Source: CAD feature listing. Evaluate the final solid. Frame: model axes, mm. Coordinates: 2 decimals unless noted, no trailing zeros. Order: outer loops, then holes, each group sorted by start corner. A loop starts at its lowest first (then second) coordinate and runs counter-clockwise, first axis right, second up.
```python
from build123d import *

# Parameters (mm, degrees)
F1_DEPTH    = 3
F2_T1_DEPTH = 3


# Not quite as in the source:
# - a fillet or chamfer that OpenCascade refuses, or shapes differently, is made with other operations: its cross-section is extruded or revolved along the edge and cut away or added


with BuildPart() as f1:
    # F0 (on Front) → F1 (new body)
    with BuildSketch(Plane.XZ):
        with BuildLine():
            Line((-12.6923788449, -38.0739606037), (-14.2292520278, -43.8096494069))
            ThreePointArc((-14.2292520278, -43.8096494069), (-12.3693152355, -44.4080485447), (-10.4843489922, -44.9221970263))
            ThreePointArc((-10.4843489922, -44.9221970263), (-10.6097140662, -41.870019803), (-7.9435705793, -43.3610533745))
            ThreePointArc((-7.9435705793, -43.3610533745), (-8.4561337122, -44.5984902415), (-9.6935705793, -45.1110533745))
            ThreePointArc((-9.6935705793, -45.1110533745), (-7.8201224186, -45.4967770693), (-5.9315086401, -45.7996446565))
            Line((-5.9315086401, -45.7996446565), (-4.35, -39.8973740589))
            ThreePointArc((-4.35, -39.8973740589), (-8.5698237047, -39.2081761686), (-12.6923788449, -38.0739606037))
        make_face()
        with BuildLine():
            Line((-14.2292520278, -43.8096494069), (-14.9257175554, -46.4088941417))
            ThreePointArc((-14.9257175554, -46.4088941417), (-10.8052141087, -47.537457316), (-6.6017256924, -48.3009287476))
            Line((-6.6017256924, -48.3009287476), (-5.9315086401, -45.7996446565))
            ThreePointArc((-5.9315086401, -45.7996446565), (-7.8201224186, -45.4967770693), (-9.6935705793, -45.1110533745))
            ThreePointArc((-9.6935705793, -45.1110533745), (-10.1000792565, -45.063184596), (-10.4843489922, -44.9221970263))
            ThreePointArc((-10.4843489922, -44.9221970263), (-12.3693152355, -44.4080485447), (-14.2292520278, -43.8096494069))
        make_face()
        with BuildLine():
            ThreePointArc((14.9257175554, -46.4088941417), (39.3966447228, -28.7135313848), (48.75, 0))
            ThreePointArc((48.75, 0), (-28.7135313848, 39.3966447228), (-14.9257175554, -46.4088941417))
            Line((-14.9257175554, -46.4088941417), (-14.2292520278, -43.8096494069))
            ThreePointArc((-14.2292520278, -43.8096494069), (-25.1843873236, 32.6155595225), (43.434381424, -2.7721802304))
            ThreePointArc((43.434381424, -2.7721802304), (35.3877397529, -27.956567554), (14.2292520278, -43.8096494069))
            Line((14.2292520278, -43.8096494069), (14.9257175554, -46.4088941417))
        make_face()
        with BuildLine():
            ThreePointArc((10.4843489922, -44.9221970263), (12.3693152355, -44.4080485447), (14.2292520278, -43.8096494069))
            Line((14.2292520278, -43.8096494069), (12.6923788449, -38.0739606037))
            ThreePointArc((12.6923788449, -38.0739606037), (8.5698237047, -39.2081761686), (4.35, -39.8973740589))
            Line((4.35, -39.8973740589), (5.9315086401, -45.7996446565))
            ThreePointArc((5.9315086401, -45.7996446565), (7.8201224186, -45.4967770693), (9.6935705793, -45.1110533745))
            ThreePointArc((9.6935705793, -45.1110533745), (8.4561337122, -42.1236165074), (11.4435705793, -43.3610533745))
            ThreePointArc((11.4435705793, -43.3610533745), (11.1846041508, -44.2771968614), (10.4843489922, -44.9221970263))
        make_face()
        with BuildLine():
            ThreePointArc((6.6017256924, -48.3009287476), (10.8052141087, -47.537457316), (14.9257175554, -46.4088941417))
            Line((14.9257175554, -46.4088941417), (14.2292520278, -43.8096494069))
            ThreePointArc((14.2292520278, -43.8096494069), (12.3693152355, -44.4080485447), (10.4843489922, -44.9221970263))
            ThreePointArc((10.4843489922, -44.9221970263), (10.1000792565, -45.063184596), (9.6935705793, -45.1110533745))
            ThreePointArc((9.6935705793, -45.1110533745), (7.8201224186, -45.4967770693), (5.9315086401, -45.7996446565))
            Line((5.9315086401, -45.7996446565), (6.6017256924, -48.3009287476))
        make_face()
    extrude(amount=F1_DEPTH)

    # F2: fillet of radius 5.9832263303 on 2 edges, made by hand

    # F2_s2 → F2_t1 (join)
    with BuildSketch(Plane.XZ):
        with BuildLine():
            ThreePointArc((21.0114203914, -40.7862000497), (16.2624097338, -41.2381768967), (12.6923788449, -38.0739606037))
            Line((12.6923788449, -38.0739606037), (12.5838858344, -38.124446895))
            ThreePointArc((12.5838858344, -38.124446895), (13.3452283796, -40.9727764638), (14.113664971, -43.8406208654))
            Line((14.113664971, -43.8406208654), (14.2684545363, -43.9227102855))
            ThreePointArc((14.2684545363, -43.9227102855), (17.7337895054, -42.5524219145), (21.0693082118, -40.8909311299))
            Line((21.0693082118, -40.8909311299), (21.0114203914, -40.7862000497))
        make_face()
        with BuildLine():
            ThreePointArc((-12.6923788449, -38.0739606037), (-16.2624097338, -41.2381768967), (-21.0114203914, -40.7862000497))
            Line((-21.0114203914, -40.7862000497), (-21.0693082118, -40.8909311299))
            ThreePointArc((-21.0693082118, -40.8909311299), (-17.7337895054, -42.5524219145), (-14.2684545363, -43.9227102855))
            Line((-14.2684545363, -43.9227102855), (-14.113664971, -43.8406208654))
            ThreePointArc((-14.113664971, -43.8406208654), (-13.3452283796, -40.9727764638), (-12.5838858345, -38.124446895))
            Line((-12.5838858345, -38.124446895), (-12.6923788449, -38.0739606037))
        make_face()
    extrude(amount=F2_T1_DEPTH)


solid = f1.part
```
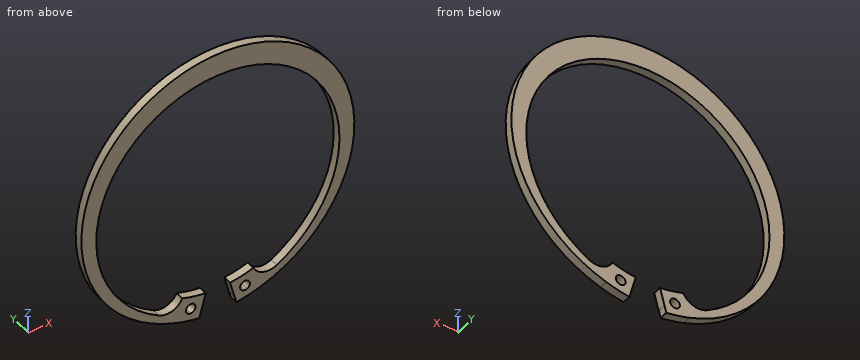
1. Material intervals for line 1 along X through (y, z) = (-1.6, 30); line 2 along Z through (x, y) = (23, -0.25); line 3 along X through (y, z) = (-0.8, 34.5), sorted ascending.
2. Section query C-C, the plane x = 32.5. Output: boundary loops of the cut face in (y, z), plus the area to 3 significant figures.
3. Section query B-B, the plane z = 20. Output: boundary loops of the cut face in (x, y), plus the area to 3 significant figures.
4. Section query D-D, the plane x = 0. Output: boundary loops of the cut face in (y, z).
5. Section query A-A, the plane y = -1.8. Output: boundary loops of the cut face in (x, z).
6. Contact query for flat-ended pins moving along their axis: P1, Ø1, axis at x = 18, y = -1, coming from the +Z side; P2, Ø1.5, axis at x = -36.5, y = -1.5, coming from the -Z side. Output: stop coordinate, or through.
Answer key:
1. line 1: x = -38.43 to -28.5, 28.5 to 38.43
1. line 2: z = -42.98 to -39.62, 34.07 to 42.98
1. line 3: x = -34.44 to -22.3, 22.3 to 34.44
2. outline: (-3, -36.34) - (0, -36.34) - (0, -31.59) - (-3, -31.59) - close; (-3, 26.04) - (0, 26.04) - (0, 36.34) - (-3, 36.34) - close
2. area: 45.1 mm2
3. outline: (-44.46, -3) - (-36.99, -3) - (-36.99, 0) - (-44.46, 0) - close; (36.99, -3) - (44.46, -3) - (44.46, 0) - (36.99, 0) - close
3. area: 44.8 mm2
4. outline: (-3, 40.66) - (0, 40.66) - (0, 48.75) - (-3, 48.75) - close
5. outline: (-21.01, -40.79) arc R43.43 cw (long way) to (21.01, -40.79) arc R5.98 cw to (12.69, -38.07) arc R40.13 cw to (4.35, -39.9) - (6.6, -48.3) arc R48.75 ccw (long way) to (-6.6, -48.3) - (-4.35, -39.9) arc R40.13 cw to (-12.69, -38.07) arc R5.98 cw to start; hole circle Ø3.5 at (-9.69, -43.36); hole circle Ø3.5 at (9.69, -43.36)
6. P1: stops at z = 45.5
6. P2: stops at z = -33.14
